```python
from build123d import *


with BuildPart() as f2:
    # F2: sweep along a path in F1
    with BuildLine(Plane.XY) as f2_path:
        Line((0, -10), (200, -10))
        Line((200, -10), (200, 490))
        Line((200, 490), (-200, 490))
        Line((-200, 490), (-200, -10))
        Line((-200, -10), (0, -10))
    # F0 (on Right) → F2 (sweep)
    with BuildSketch(Plane.YZ):
        Polygon((0, -1), (0, 0), (-10, 0), (-10, -20), (-20, -20), (-20, -21), (-9, -21), (-9, -1), align=None)
    sweep(path=f2_path.line, transition=Transition.RIGHT)


solid = f2.part
```
Can you work these out from the model? Positions are in its coordinate system, mm. A direction names the side the tool comes from. Round coordinates to 2 decimals unless told otherwise and drop trailing zeros. Loops run counter-clockwise (first coordinate to the right, second up) from the corner with the lowest first, then second, coordinate; pieces in that order, holes last. Notation, with made-up numbers: (35.5, -39.75) -> (68.5, -39.75) arc R22 ccw to (68.5, -28.75) -> close; hole circle Ø8 at (-2, 21.25). An arc over 180 degrees is marked (long way). One line per item, written item: value. Start each with the question number.
1. For faces 5 (the flat face through (200, 244, -10)), 6 (the flat face through (-3, 489, -11)), 7 (the flat face through (-200, 236, -10)), which set-ups out of +Z, -Z, +X, -X, +Y, -Y let a thin tool reach every point of the face, with its end or its side?
2. If we mould it in two halves opening along Y, with no side actions, what happens to faces 1 (the flat face through (1, 481, -1)), 2 (the flat face through (-3, 490, -10)), 3 (the flat face through (3, -10, -10)), 4 (the flat face through (-1, 482, 0))? For each: pulls with the +Y half, pulls with the -Y half, needs draft (parallel to the pull), parting line crosses it, or undercut.
3. For pin 1 (0.5 mm diameter, centred on x = 78.5, z = -0.5, fed in from -Y); pin 2 (0.8 mm diameter, centred on y = 306, z = -0.5, fed in from +X); pin 3 (6 mm diameter, centred on x = -10.5, z = -8.5, fed in from +Y), each with a flat end and sliding along its axis, tell me the tip position at first contact or that it passes through.
4. If we section it at B-B, the plane z = -4.75: Write out the boundary of the cut face in (x, y).
5. If I drill on probe 1 along X at (y, z) = (76, -16.5); probe 2 along Y at (x, z) = (51.5, -12.5); probe 3 along Z at (x, y) = (193, 94.5), over which ranges is the centre line in solid material (lowest first)?
6. If we section it at A-A, the plane y = 41: Write out the boundary of the cut face in (x, z), then the cut area to 3 significant figures.
7. If we section it at C-C, the plane x = -125: Write out the boundary of the cut face in (y, z).
Calculated:
1. face 5: +Z, +X, +Y, -Y
1. face 6: -Z
1. face 7: +Z, -X, +Y, -Y
2. face 1: undercut
2. face 2: pulls with the +Y half
2. face 3: pulls with the -Y half
2. face 4: needs draft
3. pin 1: stops at y = -10
3. pin 2: stops at x = 200
3. pin 3: stops at y = 490
4. outline: (-200, -10) -> (200, -10) -> (200, 490) -> (-200, 490) -> close; hole (-199, -9) -> (199, -9) -> (199, 489) -> (-199, 489) -> close
5. probe 1: x = -200 to -199, 199 to 200
5. probe 2: y = -10 to -9, 489 to 490
5. probe 3: z = -1 to 0
6. outline: (-210, -21) -> (-199, -21) -> (-199, -1) -> (-190, -1) -> (-190, 0) -> (-200, 0) -> (-200, -20) -> (-210, -20) -> close; (190, -1) -> (199, -1) -> (199, -21) -> (210, -21) -> (210, -20) -> (200, -20) -> (200, 0) -> (190, 0) -> close
6. area: 80.0 mm²
7. outline: (-20, -21) -> (-9, -21) -> (-9, -1) -> (0, -1) -> (0, 0) -> (-10, 0) -> (-10, -20) -> (-20, -20) -> close; (480, -1) -> (489, -1) -> (489, -21) -> (500, -21) -> (500, -20) -> (490, -20) -> (490, 0) -> (480, 0) -> close
